Geometry check sheet. Reference: the model listing, model coordinates, mm. A direction names the side the tool comes from. Coordinates: 2 decimals unless noted, no trailing zeros. Write each loop counter-clockwise with the first axis right and the second up, starting at its lowest first coordinate (ties: lowest second). Pieces come first, ordered by that corner, then holes. Notation, with made-up numbers: (76.5, 84.5) -> (81.5, 84.5) arc R27 cw to (81.5, 101.5) -> close; hole circle Ø1 at (6, -13.5). An arc over 180 degrees is marked (long way). Answer in a Markdown table with one row per item. Add a question column.
1. Set-up check for faces 4 (the flat face through (17, -43, -5)), 5 (the flat face through (0, -5, -5)), 6 (the flat face through (0, -21, 1.5)), 7 (the cylindrical face through (-0.24, -15.19, -1.86)): record each of +Z, -Z, +X, -X, +Y, -Y from which the full face is reachable in a straight line by a thin tool's end or side.
2. Cross-section at C-C on y = -22. Record the cut outline in (x, z), and give its area (3 significant figures).
3. Depth check by flat-ended pin: P1, Ø4, axis at y = 0, z = 0, coming from the -X side; P2, Ø1.5, axis at x = 7.5, y = -16, coming from the +Z side; P3, Ø3, axis at x = 1.5, y = -3.5, coming from the -Z side; P4, Ø1.5, axis at x = 5.5, z = 1, coming from the -Y side. Enter the tip coordinate at first touch or a pass-through.
4. Scan lines: L1, parallel to Y at x = 3.5, z = 1; L2, parallel to Z at x = 1, y = 0; L3, parallel to Z at x = -12, y = -22. Record each from-to range of solid material in increasing order. Write a range as from..to.
5. Cross-section at B-B on z = -4. Record the cut outline in (x, y), and give its area (3 significant figures).
6. Mould release check, pull along Y, two halves, no side actions. Record for faces 1 (the flat face through (0, -93.87, 17)), 2 (the cylindrical face through (0.24, -74.89, -5.78)), 3 (the cylindrical face through (-0.238, -76.547, -9.778)): pulls with the +Y half, pulls with the -Y half, needs draft (parallel to the pull), parting line crosses it, or undercut.
7. Cross-section at D-D on z = 16.5. Record the cut outline in (x, y).
8. Cross-section at A-A on x = 15. Record the cut outline in (y, z), and give its area (3 significant figures).
```python
from build123d import *

# Parameters (mm, degrees)
F0_R     = 1.75
F1_DEPTH = 17.5
F3_DEPTH = 35
F4_R     = 3
F5_DEPTH = 0.5
F6_DEPTH = 0.5


with BuildPart() as f1:
    # F0 (on Right) → F1 (new body, symmetric)
    with BuildSketch(Plane.YZ):
        with BuildLine():
            Line((-5.2303039929, -1.5), (-4.7696960071, -1.5))
            ThreePointArc((-4.7696960071, -1.5), (5, 0), (-4.7696960071, 1.5))
            Line((-4.7696960071, 1.5), (-37.5, 1.5))
            Line((-37.5, 1.5), (-45, -6))
            Line((-45, -6), (-75, -6))
            Line((-75, -6), (-93.8700576851, 12.8700576851))
            Line((-93.8700576851, 12.8700576851), (-93.8700576851, 20.3700576851))
            ThreePointArc((-93.8700576851, 20.3700576851), (-95.8700576851, 22.3700576851), (-97.8700576851, 20.3700576851))
            Line((-97.8700576851, 20.3700576851), (-97.8700576851, 11.2132034356))
            Line((-97.8700576851, 11.2132034356), (-76.6568542495, -10))
            Line((-76.6568542495, -10), (-43.3431457505, -10))
            Line((-43.3431457505, -10), (-34.8431457505, -1.5))
            Line((-34.8431457505, -1.5), (-14.7696960071, -1.5))
            ThreePointArc((-14.7696960071, -1.5), (-10, -5), (-5.2303039929, -1.5))
        make_face()
        Circle(F0_R, mode=Mode.SUBTRACT)
    extrude(amount=F1_DEPTH, both=True)

    # F2 (on face) → F3 (join, through all)
    with BuildSketch(Plane.YZ.offset(17.5)):
        with BuildLine():
            ThreePointArc((-5.2303039929, -1.5), (-7.0419601085, -4.0311288741), (-10, -5))
            Line((-10, -5), (0, -5))
            ThreePointArc((0, -5), (-2.9580398915, -4.0311288741), (-4.7696960071, -1.5))
            Line((-4.7696960071, -1.5), (-5.2303039929, -1.5))
        make_face()
    extrude(amount=-F3_DEPTH)

    # F4
    f4_edges = [f1.edges().sort_by_distance(p)[0] for p in [
        (0, -4.769696, 1.5),
        (0, -14.769696, -1.5),
        (0, -75, -6),
        (0, -76.656854, -10),
        (0, -43.343146, -10),
        (0, -34.843146, -1.5),
        (0, -45, -6),
        (0, -37.5, 1.5),
        (0, -97.870058, 11.213203),
        (0, -93.870058, 12.870058),
    ]]
    fillet(f4_edges, radius=F4_R)

    # F5 (cut): a face of the model
    f5_faces = [f1.faces().sort_by_distance(p)[0] for p in [
        (17.5, -96.7916296902, 16.4129509039),
    ]]
    extrude(f5_faces, amount=-F5_DEPTH, mode=Mode.SUBTRACT)

    # F6 (cut): a face of the model
    f6_faces = [f1.faces().sort_by_distance(p)[0] for p in [
        (-17.5, -96.7916296902, 16.4129509039),
    ]]
    extrude(f6_faces, amount=-F6_DEPTH, mode=Mode.SUBTRACT)


solid = f1.part
```
Results found:
| question | item | result |
|---|---|---|
| 1 | face 4 | +Z, -Z, +X, +Y, -Y |
| 1 | face 5 | -Z, +X, -X, +Y |
| 1 | face 6 | +Z, +X, -X |
| 1 | face 7 | -Z, +X, -X |
| 2 | outline | (-17, -1.5) -> (17, -1.5) -> (17, 1.5) -> (-17, 1.5) -> close |
| 2 | area | 102 mm^2 |
| 3 | P1 | stops at x = -17 |
| 3 | P2 | stops at z = 1.5 |
| 3 | P3 | stops at z = -5 |
| 3 | P4 | stops at y = -88.41 |
| 4 | L1 | y = -87.66..-82, -37.92..-1.44, 1.44..4.9 |
| 4 | L2 | z = -5..-1.75, 1.75..5 |
| 4 | L3 | z = -1.5..1.5 |
| 5 | outline | (-17, -82.66) -> (17, -82.66) -> (17, -77) -> (-17, -77) -> close; (-17, -43) -> (17, -43) -> (17, -37.34) -> (-17, -37.34) -> close; (-17, -13) -> (17, -13) -> (17, 3) -> (-17, 3) -> close |
| 5 | area | 929 mm^2 |
| 6 | face 1 | pulls with the +Y half |
| 6 | face 2 | undercut |
| 6 | face 3 | pulls with the -Y half |
| 7 | outline | (-17, -97.87) -> (17, -97.87) -> (17, -93.87) -> (-17, -93.87) -> close |
| 8 | outline | (-97.87, 12.46) arc R3 ccw to (-96.99, 10.33) -> (-77.54, -9.12) arc R3 ccw to (-75.41, -10) -> (-44.59, -10) arc R3 ccw to (-42.46, -9.12) -> (-35.72, -2.38) arc R3 cw to (-33.6, -1.5) -> (-16.61, -1.5) arc R3 cw to (-14.13, -2.81) arc R5 ccw to (-10, -5) -> (0, -5) arc R5 ccw (long way) to (-4.13, 2.81) arc R3 cw to (-6.61, 1.5) -> (-36.26, 1.5) arc R3 ccw to (-38.38, 0.62) -> (-44.12, -5.12) arc R3 cw to (-46.24, -6) -> (-73.76, -6) arc R3 cw to (-75.88, -5.12) -> (-92.99, 11.99) arc R3 cw to (-93.87, 14.11) -> (-93.87, 20.37) arc R2 ccw to (-97.87, 20.37) -> close; hole circle Ø3.5 at (0, 0) |
| 8 | area | 524 mm^2 |
